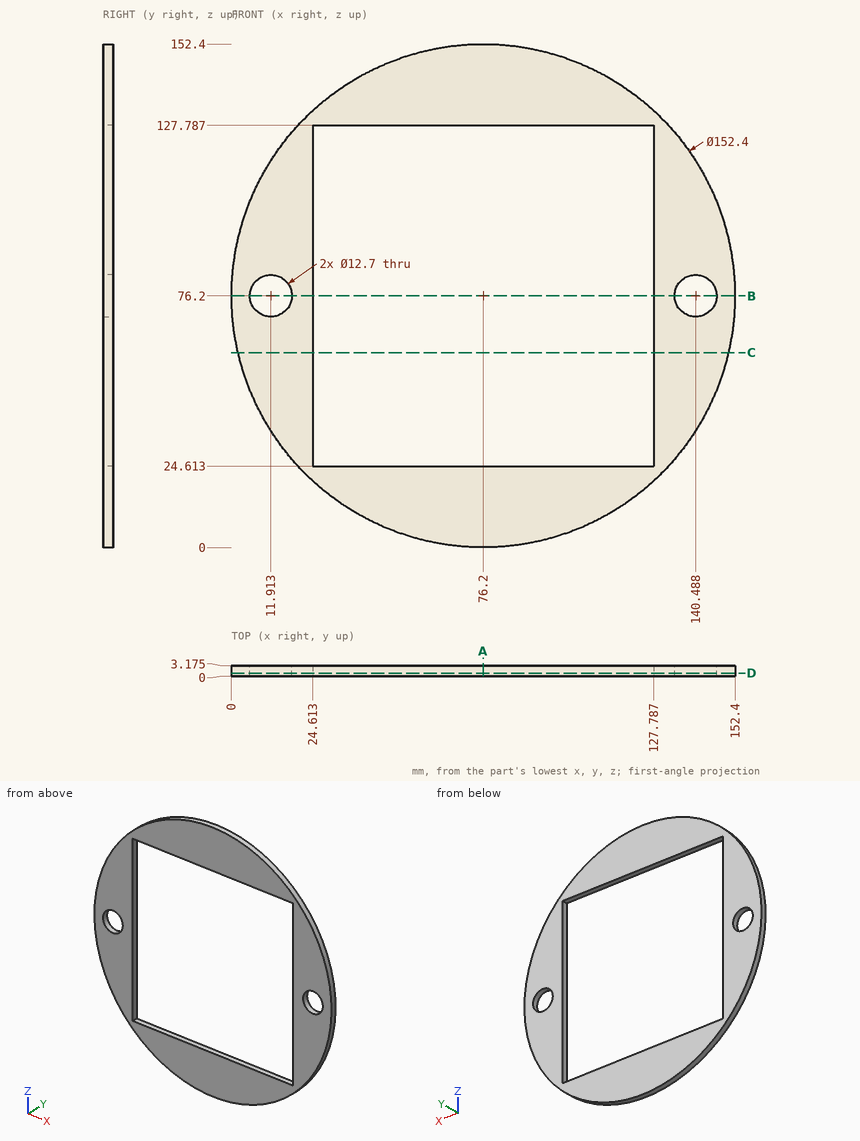
Design review of the part shown in the three views and the two pictorial views. Dimensions are in mm from the part's minimum x, y and z. Give positions to 0.01 mm unless a question says otherwise; leave off trailing zeros. Loops run counter-clockwise (first coordinate to the right, second up) from the corner with the lowest first, then second, coordinate; pieces in that order, holes last. Notation, with made-up numbers: M 11.5,-16 L 34.5,-16 A20 cw 34.5,3 Z; hole C 40.25,-21.5 d7. An arc over 180 degrees is marked long. Answer as a JSON object with one key per item and string values. Group by question number.
Q1. Add section C-C on z = 59. Give the boundary of the cut face in (x, y) (1 decimal).
Q2. Add section D-D on y = 0.9. Give the boundary of the cut face in (x, z), and give its area (3 significant figures).
Q3. Add section A-A on x = 76.2. Give the boundary of the cut face in (y, z) (1 decimal).
Q4. Add section B-B on z = 76.2. Give the boundary of the cut face in (x, y) (1 decimal).
Q5. Insertion check: P1, Ø1, axis at x = 128.5, y = 1, coming from the +Z side (1 decimal); P2, Ø1, axis at y = 2, z = 92, coming from the -X side; P3, Ø1.6, axis at y = 1.5, z = 82, coming from the -X side. Each pin has a flat end and moves straight along its axis. Give the tip position at first contact, or say it passes through.
Q6. For probe 1 along X at (y, z) = (0.85, 76.2); probe 2 along X at (y, z) = (1.6, 71.5) (1 decimal); probe 3 along Z at (x, y) = (49, 1.3), list the stretches that pass through material, from the lowest coordinate up. Write a range as [from, to].
Checked values:
{
 "1": {"outline": "M 2,0 L 24.6,0 L 24.6,3.2 L 2,3.2 Z; M 127.8,0 L 150.4,0 L 150.4,3.2 L 127.8,3.2 Z"},
 "2": {"outline": "C 76.2,76.2 d152.4; hole C 11.91,76.2 d12.7; hole M 24.61,24.61 L 127.79,24.61 L 127.79,127.79 L 24.61,127.79 Z; hole C 140.49,76.2 d12.7", "area": "7,340 mm²"},
 "3": {"outline": "M 0,0 L 3.2,0 L 3.2,24.6 L 0,24.6 Z; M 0,127.8 L 3.2,127.8 L 3.2,152.4 L 0,152.4 Z"},
 "4": {"outline": "M 0,0 L 5.6,0 L 5.6,3.2 L 0,3.2 Z; M 18.3,0 L 24.6,0 L 24.6,3.2 L 18.3,3.2 Z; M 127.8,0 L 134.1,0 L 134.1,3.2 L 127.8,3.2 Z; M 146.8,0 L 152.4,0 L 152.4,3.2 L 146.8,3.2 Z"},
 "5": {"P1": "z = 132.1", "P2": "x = 1.55", "P3": "x = 0.16"},
 "6": {"probe 1": "[0, 5.56], [18.26, 24.61], [127.79, 134.14], [146.84, 152.4]", "probe 2": "[0.1, 7.6], [16.2, 24.6], [127.8, 136.2], [144.8, 152.3]", "probe 3": "[5.02, 24.61], [127.79, 147.38]"}
}
